Autodesk Inventor part; units mm, degrees
ref_plane "YZ Plane" through (0, 0, 0) normal (1, 0, 0) x (0, 1, 0)
ref_plane "XZ Plane" through (0, 0, 0) normal (0, 1, 0) x (-1, 0, 0)
ref_plane "XY Plane" through (0, 0, 0) normal (0, 0, 1) x (1, 0, 0)
sketch "Sketch1" plane through (0, 0, 0) normal (0, 1, 0) x (-1, 0, 0)
  line L0 (60, -40) -> (-60, -40)
  line L1 (-60, -40) -> (-60, 40)
  line L2 (-60, 40) -> (60, 40)
  line L3 (60, 40) -> (60, -40)
  point P0 (0, 0)
  dimension "d0" = 80
  dimension "d1" = 120
  dimension "d2" = 40
  dimension "d3" = 60
extrude "Extrusion1" add sketch "Sketch1" along normal blind 2
sketch "Sketch2" plane through (0, 2, 0) normal (0, 1, 0) x (1, 0, 0)
  line L0 (60, 40) -> (-60, 40)
  line L1 (60, -40) -> (60, 40)
  line L2 (-60, 40) -> (60, 40)
  line L3 (60, 40) -> (60, -40)
  line L4 (60, -40) -> (-60, -40)
  line L5 (-60, -40) -> (-60, 40)
  line L6 (-58, 38) -> (58, 38)
  line L7 (58, 38) -> (58, -38)
  line L8 (58, -38) -> (-58, -38)
  line L9 (-58, -38) -> (-58, 38)
  arc A0 (-50, -34) -> (-54, -30) centre (-54, -34) ccw
  line L10 (-54, -30) -> (-58, -30)
  line L11 (-50, -34) -> (-50, -38)
  line L12 (0, 4.5233) -> (0, -3.3512)
  line L13 (-2.8256, 0) -> (3.7968, 0)
  arc A1 (-54, 30) -> (-50, 34) centre (-54, 34) ccw
  line L14 (-54, 30) -> (-58, 30)
  line L15 (-50, 34) -> (-50, 38)
  arc A2 (54, -30) -> (50, -34) centre (54, -34) ccw
  line L16 (54, -30) -> (58, -30)
  line L17 (50, -34) -> (50, -38)
  line L18 (54, 30) -> (58, 30)
  arc A3 (50, 34) -> (54, 30) centre (54, 34) ccw
  line L19 (50, 34) -> (50, 38)
  circle A4 centre (-54, -34) radius 2.5
  circle A5 centre (-54, 34) radius 2.5
  circle A6 centre (54, -34) radius 2.5
  circle A7 centre (54, 34) radius 2.5
  point P0 (0, 0)
  dimension "d6" = 2
  dimension "d7" = 2
  dimension "d8" = 2
  dimension "d9" = 2
  dimension "d29" = 8
  dimension "d30" = 4
  dimension "d31" = 4
  dimension "d32" = 5
  dimension "d35" = 68
  dimension "d38" = 108
extrude "Extrusion2" add sketch "Sketch2" along normal blind 25 contours L1 L4 L5 L0 | L6 L15 A1 L14 L9 | L6 L7 L18 A3 L19 | L10 A0 L11 L8 L9 | L7 L8 L17 A2 L16
sketch "Sketch3" plane through (-60, 0, 40) normal (0, 0, 1) x (1, 0, 0)
  line L0 (15, 22) -> (75, 22)
  line L1 (75, 22) -> (75, 7)
  line L2 (75, 7) -> (15, 7)
  line L3 (15, 7) -> (15, 22)
  line L4 (10, 2) -> (110, 2)
  line L5 (0, 0) -> (0, 27)
  line L6 (85, 17) -> (94, 17)
  line L7 (94, 17) -> (94, 7)
  line L8 (94, 7) -> (85, 7)
  line L9 (85, 7) -> (85, 17)
  line L10 (99, 22) -> (109, 22)
  line L11 (109, 22) -> (109, 7)
  line L12 (109, 7) -> (99, 7)
  line L13 (99, 7) -> (99, 22)
  circle A0 centre (89.5, 22) radius 1.5
  point P0 (60, 0)
  point P1 (2, 2)
  point P2 (118, 2)
  point P3 (89.5, 7)
  point P4 (89.5, 17)
  dimension "d12" = 60
  dimension "d13" = 15
  dimension "d14" = 5
  dimension "d15" = 15
  dimension "d16" = 9
  dimension "d17" = 10
  dimension "d18" = 10
  dimension "d19" = 5
  dimension "d20" = 10
  dimension "d21" = 15
  dimension "d22" = 5
  dimension "d23" = 5
  dimension "d24" = 3
  dimension "d25" = 5
  dimension "d26" = 4.5
extrude "Extrusion3" cut sketch "Sketch3" against normal blind 25
fillet "Fillet1" radius 4 4 edges at (-60, 13.5, 40) (60, 13.5, 40) (60, 13.5, -40) (-60, 13.5, -40)
equation "\"d0\" = 0.666667 * d1"
equation "\"d7\" = d6"
equation "\"d8\" = d6"
equation "\"d9\" = d6"
equation "\"d30\" = 0.5 * d29"
equation "\"d31\" = d30"
equation "\"d22\" = d19"
equation "\"d26\" = 0.5 * d16"
properties part number "housing_base"
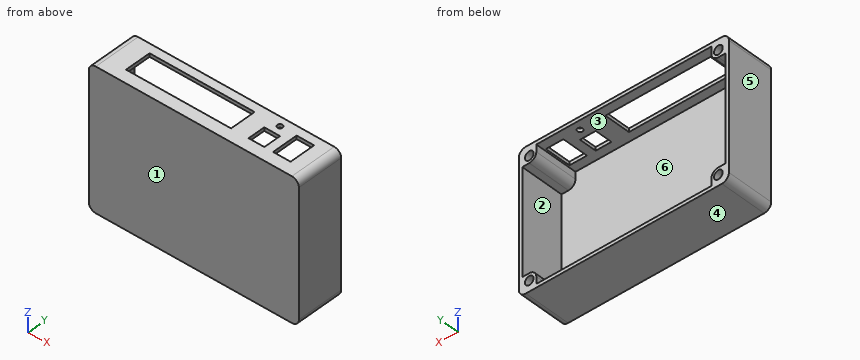
Can you work these out from the model? Positions are in its coordinate system, mm. Face numbers are marked on the shaded views. A direction names the side the tool comes from. Coordinates: 2 decimals unless noted, no trailing zeros. Write each loop counter-clockwise with the first axis right and the second up, starting at its lowest first coordinate (ties: lowest second). Pieces come first, ordered by that corner, then holes. Notation, with made-up numbers: M 42,20 L 70,20 A23 ccw 70,46 Z; hole C 48,-30 d11. An arc over 180 degrees is marked long. Use one line per item in the form item = value.
Q1. If we section it at D-D (z = -12.5): Write out the boundary of the cut face in (x, y), then the cut area to 3 significant figures.
Model answer:
outline = M -60,0 L 60,0 L 60,27 L 58,27 L 58,2 L -58,2 L -58,27 L -60,27 Z
area = 340 mm^2
Q2. If we section it at A-A (x = -36): Write out the boundary of the cut face in (y, z), then the cut area to 3 significant figures.
Model answer:
outline = M 0,-40 L 27,-40 L 27,-38 L 2,-38 L 2,38 L 7,38 L 7,40 L 0,40 Z; M 22,38 L 27,38 L 27,40 L 22,40 Z
area = 230 mm^2
Q3. For the marked faces 1 and 2, which set-ups out of +Z, -Z, +X, -X, +Y, -Y let a thin tool reach every point of the face, with its end or its side?
Model answer:
face_1 = +Z, -Z, +X, -X, -Y
face_2 = +Y
Q4. If we section it at C-C (y = 25.25): Write out the boundary of the cut face in (x, z).
Model answer:
outline = M -60,-36 A4 ccw -56,-40 L 56,-40 A4 ccw 60,-36 L 60,36 A4 ccw 56,40 L -56,40 A4 ccw -60,36 Z; hole M -58,-30 L -54,-30 A4 cw -50,-34 L -50,-38 L 50,-38 L 50,-34 A4 cw 54,-30 L 58,-30 L 58,30 L 54,30 A4 cw 50,34 L 50,38 L -50,38 L -50,34 A4 cw -54,30 L -58,30 Z; hole C -54,-34 d5; hole C -54,34 d5; hole C 54,-34 d5; hole C 54,34 d5
Q5. For P1, Ø2, axis at x = -16, y = 20.5, coming from the +Z side; P2, Ø1.5, axis at x = 53, z = -34, coming from the +Y side; P3, Ø1.6, axis at y = 11, z = 39, coming from the +X side, each with a flat end and sliding along its axis, tell me the tip position at first contact or that it passes through.
Model answer:
P1 = -38
P2 = 2
P3 = 59.34
Q6. I need wall thicknesses on line 1 along X through (y, z) = (19, 34); line 2 along Z through (x, y) = (54, 17); line 3 along X through (y, z) = (25.75, -21.5). Which ranges of each line are inside material? Lowest first, please. Write a range as from..to.
Model answer:
line_1 = -60..-56.5, -51.5..-50, 50..51.5, 56.5..60
line_2 = -40..-36.5, -31.5..-30, 30..31.5, 36.5..40
line_3 = -60..-58, 58..60
Q7. We'd pull the mould along Z, two halves only. Please class the marked faces 3, 4, 5 and 6: +Z half, -Z half, draft (parallel to the pull), parting line (faces both ways), or undercut.
Model answer:
face_3 = undercut
face_4 = -Z half
face_5 = draft
face_6 = undercut
Q8. If we section it at B-B (x = 29.5): Write out the boundary of the cut face in (y, z).
Model answer:
outline = M 0,-40 L 27,-40 L 27,-38 L 2,-38 L 2,38 L 7,38 L 7,40 L 0,40 Z; M 17,38 L 20.5,38 L 20.5,40 L 17,40 Z; M 23.5,38 L 27,38 L 27,40 L 23.5,40 Z
